Read the model definition and answer for the solid it produces. Units are mm, in the model's axes. A direction names the side the tool comes from. Coordinates: 2 decimals unless noted, no trailing zeros. Write each loop counter-clockwise with the first axis right and the second up, starting at its lowest first coordinate (ties: lowest second). Pieces come first, ordered by that corner, then holes. Notation, with made-up numbers: (75, 25) -> (130, 25) arc R7 ccw to (130, 32) -> close; hole circle Ø6 at (37.25, -10). An arc over 180 degrees is marked (long way). Return JSON: item names as keys, results as strings.
Autodesk Inventor part; units mm, degrees
ref_plane "YZ Plane" through (0, 0, 0) normal (1, 0, 0) x (0, 1, 0)
ref_plane "XZ Plane" through (0, 0, 0) normal (0, 1, 0) x (-1, 0, 0)
ref_plane "XY Plane" through (0, 0, 0) normal (0, 0, 1) x (1, 0, 0)
sketch "Sketch1" plane through (0, 0, 0) normal (0, 1, 0) x (-1, 0, 0)
  line L0 (0, 0) -> (67.2338, 0)
  arc A0 (76.7588, -9.525) -> (67.2338, 0) centre (67.2338, -9.525) ccw
  arc A1 (67.2338, -48.9204) -> (76.7588, -39.3954) centre (67.2338, -39.3954) ccw
  line L1 (76.7588, -9.525) -> (76.7588, -39.3954)
  line L2 (67.2338, -48.9204) -> (15.367, -48.9204)
  line L3 (15.367, -48.9204) -> (-3.6891, -67.9765)
  line L4 (0, 0) -> (-25.3962, 25.3962)
  circle A2 centre (35.2298, -16.4592) radius 1.905
  circle A3 centre (35.2298, -32.4612) radius 1.905
  circle A4 centre (67.2338, -32.4612) radius 1.905
  circle A5 centre (67.2338, -16.4592) radius 1.905
  circle A6 centre (-26.1112, -24.4602) radius 1.85
  circle A7 centre (-26.1112, 7.2898) radius 1.85
  line L5 (-25.3962, 25.3962) -> (-31.7462, 25.3962)
  line L6 (-31.7462, 25.3962) -> (-31.7462, -39.9194)
  line L7 (-31.7462, -39.9194) -> (-3.6891, -67.9765)
  circle A8 centre (0, -12.7) radius 1.85
  circle A9 centre (0, -38.1) radius 1.85
  line L8 (-3.6891, -67.9765) -> (-12.6694, -58.9962)
  circle A10 centre (-3.6891, -59.4929) radius 1.85
  circle A11 centre (-17.1882, -44.4383) radius 1.85
  dimension "d21" = 6.35
extrude "Extrusion1" add sketch "Sketch1" along normal blind 7
sketch "Sketch2" plane through (0, 7, 0) normal (0, 1, 0) x (1, 0, 0)
  line L0 (0, 0) -> (25.3962, -25.3962)
  line L1 (0, 0) -> (25.3962, -25.3962)
  line L2 (25.3962, -25.3962) -> (31.7462, -25.3962)
  line L3 (25.3962, -25.3962) -> (31.7462, -25.3962)
  line L4 (31.7462, -25.3962) -> (31.7462, 39.9194)
  line L5 (31.7462, -25.3962) -> (31.7462, 39.9194)
  line L6 (3.6891, 67.9765) -> (-15.367, 48.9204)
  line L7 (31.7462, 39.9194) -> (3.6891, 67.9765)
  line L8 (3.6891, 67.9765) -> (-15.367, 48.9204)
  arc A0 (-67.2338, 48.9204) -> (-76.7588, 39.3954) centre (-67.2338, 39.3954) ccw
  line L9 (-15.367, 48.9204) -> (-67.2338, 48.9204)
  line L10 (-67.2338, 0) -> (0, 0)
  line L11 (0, 0) -> (-67.2338, 0)
  arc A1 (-67.2338, 48.9204) -> (-76.7588, 39.3954) centre (-67.2338, 39.3954) ccw
  arc A2 (-76.7588, 9.525) -> (-67.2338, 0) centre (-67.2338, 9.525) ccw
  arc A3 (-76.7588, 9.525) -> (-67.2338, 0) centre (-67.2338, 9.525) ccw
  line L12 (-76.7588, 39.3954) -> (-76.7588, 9.525)
  line L13 (-76.7588, 39.3954) -> (-76.7588, 9.525)
  circle A4 centre (3.6891, 59.4929) radius 1.85
  circle A5 centre (3.6891, 59.4929) radius 1.85
  circle A6 centre (0, 38.1) radius 1.85
  circle A7 centre (0, 38.1) radius 1.85
  circle A8 centre (17.1882, 44.4383) radius 1.85
  circle A9 centre (17.1882, 44.4383) radius 1.85
  circle A10 centre (26.1112, 24.4602) radius 1.85
  circle A11 centre (26.1112, 24.4602) radius 1.85
  circle A12 centre (26.1112, -7.2898) radius 1.85
  circle A13 centre (26.1112, -7.2898) radius 1.85
  circle A14 centre (0, 12.7) radius 1.85
  circle A15 centre (0, 12.7) radius 1.85
  circle A16 centre (-35.2298, 16.4592) radius 1.905
  circle A17 centre (-35.2298, 16.4592) radius 1.905
  circle A18 centre (-35.2298, 32.4612) radius 1.905
  circle A19 centre (-35.2298, 32.4612) radius 1.905
  circle A20 centre (-67.2338, 32.4612) radius 1.905
  circle A21 centre (-67.2338, 32.4612) radius 1.905
  circle A22 centre (-67.2338, 16.4592) radius 1.905
  circle A23 centre (-67.2338, 16.4592) radius 1.905
extrude "Extrusion2" add sketch "Sketch2" along normal blind 3
properties part number "MotorSuspension"
1. Flat-ended cylindrical pins translate along their axes: pin 1 Ø1.5 at (x, z) = (-50, 2) entering from -Y; pin 2 Ø1.5 at (x, y) = (13, 3) entering from -Z; pin 3 Ø6 at (y, z) = (7, -52) entering from +X; pin 4 Ø3 at (x, y) = (-22.5, 7) entering from +Z. Find the tip coordinate at first contact, or state that the pin passes through.
Taken from the geometry:
{"pin 1": "passes through", "pin 2": "stops at z = -59.42", "pin 3": "stops at x = 22.67", "pin 4": "stops at z = 0"}
2. The part is cut by section A-A (y = 4.5). Count the separate pieces of the cut face and the enclosed holes in it, then the cut area to 3 significant figures.
Taken from the geometry:
{"separate pieces": "1", "enclosed holes": "10", "area": "5,970 mm2"}
3. The part is cut by section B-B (z = 2.5). Determine the outline of the cut face in (x, y), then the cut area to 3 significant figures.
Taken from the geometry:
{"outline": "(2.5, 0) -> (31.75, 0) -> (31.75, 10) -> (2.5, 10) -> close", "area": "292 mm2"}
4. The part is cut by section C-C (x = -57.5). Determine the outline of the cut face in (y, z).
Taken from the geometry:
{"outline": "(0, -48.92) -> (10, -48.92) -> (10, 0) -> (0, 0) -> close"}
5. Consider L1, parallel to Z at x = -67.5, y = 5.5; L2, parallel to X at y = 4.5, z = -31; L3, parallel to Z at x = -62.5, y = 5.75. Determine where each line is inside the solid, lowest interval first.
Taken from the geometry:
{"L1": "z = -48.92 to -34.35, -30.57 to -18.35, -14.57 to 0", "L2": "x = -76.76 to -68.46, -66.01 to -36.45, -34.01 to 31.75", "L3": "z = -48.92 to 0"}
6. A tool of negligible diameter and unlimited length cuts with its end or side. For faces 1 (the face through (31.746, 5, -7)), 2 (the face through (-33, 5, 0)), from which of +Z, -Z, +X, -X, +Y, -Y can it reach the whole face along a straight path? Write none if from no direction.
Taken from the geometry:
{"face 1": "+Z, -Z, +X, +Y, -Y", "face 2": "+Z, -X, +Y, -Y"}
